Here's how the part is built. I have some questions about the finished solid (model axes, mm). A direction names the side the tool comes from. Give positions to 0.01 mm unless a question says otherwise; leave off trailing zeros. Write each loop counter-clockwise with the first axis right and the second up, starting at its lowest first coordinate (ties: lowest second). Pieces come first, ordered by that corner, then holes. Notation, with made-up numbers: M 42.25,-12.5 L 92.25,-12.5 A19 cw 92.25,-4.5 Z; hole C 39.5,39 d10. An arc over 180 degrees is marked long. Use one line per item in the form item = value. Start each with the question number.
Autodesk Fusion 360 part; units mm, degrees
sketch "Sketch1" plane through (0, 0, 0) normal (0, 1, 0) x (1, 0, 0)
  circle A0 centre (0, 0) radius 150
  dimension "d1" = 300
extrude "Extrude1" add sketch "Sketch1" along normal blind 10
fillet "Fillet1" radius 4 1 edges at (-139.8491, 10, 54.2423)
fillet "Fillet2" radius 4 1 edges at (-139.8491, 0, 54.2423)
sketch "Sketch2" plane through (0, 0, 0) normal (0, -1, 0) x (1, 0, 0)
  circle A0 centre (0, 0) radius 146
sketch "Sketch3" plane through (0, 0, 0) normal (0, 1, 0) x (1, 0, 0)
  circle A0 centre (0, 0) radius 1.555
  dimension "d12" = 3.11
extrude "Extrude2" cut sketch "Sketch3" along normal blind 11
sketch "Sketch4" plane through (0, 10, 0) normal (0, 1, 0) x (-1, 0, 0)
  circle A0 centre (0, 0) radius 1.555
  circle A1 centre (0, 0) radius 146
  line L0 (120, -40) -> (90, 40)
  line L1 (90, 40) -> (60, 40)
  line L2 (60, 40) -> (30, -40)
  line L3 (30, -40) -> (50, -40)
  line L4 (50, -40) -> (70, 20)
  line L5 (70, 20) -> (80, 20)
  line L6 (80, 20) -> (100, -40)
  line L7 (100, -40) -> (120, -40)
  line L8 (-30, -30) -> (-50, -30)
  arc A2 (-70, -30) -> (-50, -30) centre (-60, -30) ccw
  arc A3 (-90, -30) -> (-30, -30) centre (-60, -30) ccw
  spline S0 degree 5 poles (-70, -30) (-70.0634, -29.7236) (-70.1723, -29.1665) (-70.2819, -28.3178) (-70.3207, -27.1599) (-70.1889, -25.6686) (-69.8751, -24.1335) (-69.376, -22.5546) (-68.6884, -20.9329) (-67.8134, -19.2713) (-66.7594, -17.5764) (-65.547, -15.8596) (-64.2094, -14.1377) (-62.7845, -12.4293) (-61.3071, -10.7508) (-59.8021, -9.1139) (-58.2756, -7.5214) (-56.7101, -5.965) (-55.0757, -4.4303) (-53.3406, -2.9009) (-51.4819, -1.3633) (-49.4955, 0.189) (-47.4087, 1.7499) (-45.2741, 3.3045) (-43.1564, 4.8358) (-41.1228, 6.3305) (-39.2311, 7.7847) (-37.5194, 9.21) (-35.9935, 10.6403) (-34.6345, 12.1238) (-33.4107, 13.7116) (-32.2874, 15.4473) (-31.2375, 17.3568) (-30.2526, 19.4371) (-29.3384, 21.6635) (-28.5106, 23.9969) (-27.7898, 26.3921) (-27.1977, 28.8042) (-26.7512, 31.1975) (-26.4611, 33.5493) (-26.3334, 35.8458) (-26.3632, 37.6333) (-26.46, 38.9452) (-26.5577, 39.8069) (-26.6147, 40.2346) knots 0 0 0 0 0 0 0.025 0.05 0.075 0.1 0.125 0.15 0.175 0.2 0.225 0.25 0.275 0.3 0.325 0.35 0.375 0.4 0.425 0.45 0.475 0.5 0.525 0.55 0.575 0.6 0.625 0.65 0.675 0.7 0.725 0.75 0.775 0.8 0.825 0.85 0.875 0.9 0.925 0.95 0.975 1 1 1 1 1 1
  spline S1 degree 5 poles (-90, -30) (-90.0442, -29.7838) (-90.1209, -29.3378) (-90.2007, -28.6279) (-90.2365, -27.5994) (-90.1634, -26.1809) (-89.9721, -24.6411) (-89.6627, -23.0046) (-89.2357, -21.3104) (-88.6909, -19.6034) (-88.0272, -17.9257) (-87.2416, -16.31) (-86.328, -14.7695) (-85.2785, -13.2964) (-84.0856, -11.8706) (-82.7446, -10.4656) (-81.2559, -9.0553) (-79.6283, -7.6214) (-77.8793, -6.1572) (-76.0322, -4.6645) (-74.114, -3.1522) (-72.1524, -1.6337) (-70.1735, -0.1252) (-68.1991, 1.3564) (-66.2443, 2.796) (-64.3188, 4.1811) (-62.4289, 5.504) (-60.5798, 6.763) (-58.7772, 7.9643) (-57.0291, 9.1229) (-55.3486, 10.266) (-53.7526, 11.4282) (-52.2604, 12.6449) (-50.8915, 13.9443) (-49.6636, 15.3415) (-48.5909, 16.8301) (-47.6823, 18.3787) (-46.9432, 19.942) (-46.3762, 21.4701) (-45.982, 22.9167) (-45.7603, 24.2509) (-45.7206, 25.2167) (-45.768, 25.8818) (-45.8338, 26.299) (-45.8753, 26.5009) knots 0 0 0 0 0 0 0.025 0.05 0.075 0.1 0.125 0.15 0.175 0.2 0.225 0.25 0.275 0.3 0.325 0.35 0.375 0.4 0.425 0.45 0.475 0.5 0.525 0.55 0.575 0.6 0.625 0.65 0.675 0.7 0.725 0.75 0.775 0.8 0.825 0.85 0.875 0.9 0.925 0.95 0.975 1 1 1 1 1 1
  line L9 (-45.8753, 26.5009) -> (-90, 26.5009)
  line L10 (-90, 26.5009) -> (-90, 40)
  line L11 (-90, 40) -> (-26.6147, 40.2346)
  point P0 (-70, -24.8518)
  point P1 (-67, -18)
  point P2 (-60, -9.3422)
  point P3 (-51, -1)
  point P4 (-39, 8)
  point P5 (-32.2588, 15.5698)
  point P6 (-27.4521, 27.8408)
  point P7 (-90, -25)
  point P8 (-87.5787, -17.0448)
  point P9 (-81.7168, -9.508)
  point P10 (-70, 0)
  point P11 (-58.1016, 8.4127)
  point P12 (-50, 15)
  point P13 (-46.2103, 22.1464)
extrude "Extrude3" cut sketch "Sketch4" against normal blind 1 contours L0 L1 L2 L3 L4 L5 L6 L7 | L8 A2 A3 S0 S1 L9 L10 L11
scale "Scale1" factor 0.5 about (-120, 10, -40) bodies 1
sketch "Sketch5" plane through (0, 10, 0) normal (0, 1, 0) x (-1, 0, 0)
  line L0 (105, 0) -> (120, -40)
  line L1 (120, -40) -> (110, -40)
  line L2 (110, -40) -> (100, -10)
  line L3 (100, -10) -> (95, -10)
  line L4 (95, -10) -> (85, -40)
  line L5 (85, -40) -> (75, -40)
  line L6 (75, -40) -> (90, 0)
  line L7 (90, 0) -> (105, 0)
  line L8 (35, -35) -> (45, -35)
  arc A0 (15, -35) -> (45, -35) centre (30, -35) ccw
  spline S0 degree 5 poles (15, -35) (14.9779, -34.8919) (14.9396, -34.6689) (14.8997, -34.3139) (14.8818, -33.7997) (14.9183, -33.0904) (15.0139, -32.3206) (15.1686, -31.5023) (15.3821, -30.6552) (15.6545, -29.8017) (15.9864, -28.9629) (16.3792, -28.155) (16.836, -27.3848) (17.3607, -26.6482) (17.9572, -25.9353) (18.6277, -25.2328) (19.372, -24.5277) (20.1858, -23.8107) (21.0604, -23.0786) (21.9839, -22.3322) (22.943, -21.5761) (23.9238, -20.8169) (24.9133, -20.0626) (25.9004, -19.3218) (26.8778, -18.602) (27.8406, -17.9094) (28.7856, -17.248) (29.7101, -16.6185) (30.6114, -16.0179) (31.4854, -15.4385) (32.3257, -14.867) (33.1237, -14.2859) (33.8698, -13.6776) (34.5542, -13.0279) (35.1682, -12.3293) (35.7046, -11.585) (36.1589, -10.8107) (36.5284, -10.029) (36.8119, -9.265) (37.009, -8.5416) (37.1199, -7.8746) (37.1397, -7.3916) (37.116, -7.0591) (37.0831, -6.8505) (37.0623, -6.7495) knots 0 0 0 0 0 0 0.025 0.05 0.075 0.1 0.125 0.15 0.175 0.2 0.225 0.25 0.275 0.3 0.325 0.35 0.375 0.4 0.425 0.45 0.475 0.5 0.525 0.55 0.575 0.6 0.625 0.65 0.675 0.7 0.725 0.75 0.775 0.8 0.825 0.85 0.875 0.9 0.925 0.95 0.975 1 1 1 1 1 1
  line L9 (37.0623, -6.7495) -> (15, -6.7495)
  line L10 (15, -6.7495) -> (15, 0)
  line L11 (15, 0) -> (46.6926, 0.1173)
  spline S1 degree 5 poles (46.6926, 0.1173) (46.7212, -0.0965) (46.77, -0.5274) (46.8184, -1.1833) (46.8333, -2.0771) (46.7694, -3.2253) (46.6244, -4.4012) (46.4012, -5.5979) (46.1051, -6.804) (45.7447, -8.0015) (45.3308, -9.1683) (44.8737, -10.2814) (44.3812, -11.3216) (43.8563, -12.2763) (43.2946, -13.1442) (42.6827, -13.9381) (42.0033, -14.6798) (41.2403, -15.395) (40.3845, -16.1076) (39.4386, -16.8347) (38.4218, -17.5821) (37.363, -18.3478) (36.2956, -19.1251) (35.2523, -19.9055) (34.259, -20.6816) (33.3297, -21.4504) (32.4621, -22.2152) (31.645, -22.9825) (30.8622, -23.7607) (30.099, -24.5569) (29.3464, -25.3754) (28.6078, -26.2146) (27.8953, -27.0689) (27.2265, -27.9298) (26.6203, -28.7882) (26.0933, -29.6357) (25.6558, -30.4664) (25.312, -31.2773) (25.0624, -32.0667) (24.9055, -32.8343) (24.8397, -33.5799) (24.859, -34.1589) (24.9139, -34.5833) (24.9683, -34.8618) (25, -35) knots -1 -1 -1 -1 -1 -1 -0.975 -0.95 -0.925 -0.9 -0.875 -0.85 -0.825 -0.8 -0.775 -0.75 -0.725 -0.7 -0.675 -0.65 -0.625 -0.6 -0.575 -0.55 -0.525 -0.5 -0.475 -0.45 -0.425 -0.4 -0.375 -0.35 -0.325 -0.3 -0.275 -0.25 -0.225 -0.2 -0.175 -0.15 -0.125 -0.1 -0.075 -0.05 -0.025 0 0 0 0 0 0
  arc A1 (25, -35) -> (35, -35) centre (30, -35) ccw
  circle A2 centre (60, -20) radius 0.7775
  circle A3 centre (60, -20) radius 73
  circle A4 centre (60, -20) radius 1.555
  dimension "d18" = 3.11
extrude "Extrude4" cut sketch "Sketch5" against normal blind 11 contours A4
1) Thinking about a two-plate mould opening in Z: for faces 1 (the face through (-115.278, 7.493, 30.689)), 2 (the face through (-102, 9.5, -15)), 3 (the face through (-45, 5, -21)), which applies, released by +Z, released by -Z, zero draft, split by the parting line, or undercut?
2) Suppose I cut it at A-A, the plane y = 5.9. List the corners of the cut face in (x, z) for me (3 decimals), and give its area (3 significant figures).
3) Please list where these lines run through material, in increasing order: line 1 (Z direction, x = -60, y = 6.55) (3 decimals); line 2 (Z direction, x = -60, y = 9) (3 decimals); line 3 (Y direction, x = -86.5, z = -24.5).
4) On a 3-axis mill with a long thin cutter (end or side, diameter ignored), from which of +Z, -Z, +X, -X, +Y, -Y can I reach the whole of each face in a straight line? I mean faces 4 (the face through (-45, 10, -21)), 5 (the face through (-29.67, 9.754, -49.996)). Say none if no direction works.
5) Will these pins go through, and if not, where does the flat tip stop? P1, Ø1.5, axis at x = -116.5, y = 6.5, coming from the -Z side; P2, Ø12, axis at x = -90, z = -11, coming from the +Y side; P3, Ø1.5, axis at x = -61, y = 8.5, coming from the -Z side; P4, Ø2, axis at x = -25.5, y = 7, coming from the +Z side.
Checks:
q1.face_1 = split by the parting line
q1.face_2 = undercut
q1.face_3 = zero draft
q2.outline = C -60,-20 d149.341; hole C -60,-20 d3.11
q2.area = 17,500 mm^2
q3.line_1 = -94.949 to -21.555, -18.445 to 54.949
q3.line_2 = -94.732 to -21.555, -18.445 to 54.732
q3.line_3 = 5 to 9.5
q4.face_4 = +Z, -Z, +X, -X, +Y
q4.face_5 = +Y
q5.P1 = -70.11
q5.P2 = 10
q5.P3 = -95
q5.P4 = 47.1
